```python
from build123d import *

# Parameters (mm, degrees)
EXTRUDE_1_DEPTH           = 20
EXTRUDE_2_DEPTH           = 18.5
EXTRUDE_START             = -6.5
EXTRUDE_8_DEPTH           = 6.5
CUT_EXTRUDE_1_DEPTH       = 3
CUT_EXTRUDE_12_REACH      = 37.343
SKETCH_8_W                = 8
SKETCH_8_H                = 3
SKETCH_1_10_R             = 1.1
CUT_EXTRUDE_13_DEPTH      = 38.032676918
SKETCH_18_W               = 11.552
SKETCH_18_H               = 1
CUT_EXTRUDE_16_DEPTH      = 43.464917168
CHAMFER_1_SIZE            = 4
CHAMFER_1_SIZE2           = 2.309401077
CUT_EXTRUDE_18_REACH      = 39.033
EXTRUDE_START_2           = 3.7
EXTRUDE_9_DEPTH           = 3.7
CUT_EXTRUDE_19_DEPTH      = 11.5
CUT_EXTRUDE_19_DEPTH_BACK = 15.742
SKETCH_22_W               = 16
SKETCH_22_H               = 1.5


with BuildPart() as part:
    # 草图1 → 凸台-拉伸1 (new body)
    with BuildSketch(Plane(origin=(0, 0, 0), x_dir=(1, 0, 0), z_dir=(0, 1, 0))):
        with BuildLine():
            Line((9.493752892, 13.289712364), (-9.506247108, 13.289712364))
            ThreePointArc((-9.506247108, 13.289712364), (-11.274014061, 12.557479317), (-12.006247108, 10.789712364))
            Line((-12.006247108, 10.789712364), (-12.006247108, -10.762287636))
            ThreePointArc((-12.006247108, -10.762287636), (-11.274014061, -12.530054589), (-9.506247108, -13.262287636))
            Line((-9.506247108, -13.262287636), (9.493752892, -13.262287636))
            ThreePointArc((9.493752892, -13.262287636), (11.261519845, -12.530054589), (11.993752892, -10.762287636))
            Line((11.993752892, -10.762287636), (11.993752892, 10.789712364))
            ThreePointArc((11.993752892, 10.789712364), (11.261519845, 12.557479317), (9.493752892, 13.289712364))
        make_face()
        with BuildLine():
            Line((-9.672300027, -7.488904962), (-9.672300027, 7.483095038))
            ThreePointArc((-9.672300027, 7.483095038), (-7.197426293, 8.508221304), (-6.172300027, 10.983095038))
            Line((-6.172300027, 10.983095038), (6.159805812, 10.983095038))
            ThreePointArc((6.159805812, 10.983095038), (7.184932077, 8.508221304), (9.659805812, 7.483095038))
            Line((9.659805812, 7.483095038), (9.659805812, -7.488904962))
            ThreePointArc((9.659805812, -7.488904962), (7.184932077, -8.514031228), (6.159805812, -10.988904962))
            Line((6.159805812, -10.988904962), (-6.172300027, -10.988904962))
            ThreePointArc((-6.172300027, -10.988904962), (-7.197426293, -8.514031228), (-9.672300027, -7.488904962))
        make_face(mode=Mode.SUBTRACT)
    extrude(amount=EXTRUDE_1_DEPTH)

    # 草图3<8> → 凸台-拉伸2 (add)
    with BuildSketch(Plane(origin=(0, 0, 0), x_dir=(1, 0, 0), z_dir=(0, 1, 0))):
        with BuildLine():
            Line((-1.499580884, 4.180163842), (-6.383603139, 9.785400263))
            ThreePointArc((-6.383603139, 9.785400263), (-7.282338381, 8.426127434), (-8.699129058, 7.621110763))
            Line((-8.699129058, 7.621110763), (-3.200900077, 1.310968891))
            ThreePointArc((-3.200900077, 1.310968891), (-2.708791154, -0.002904962), (-3.200900077, -1.316778815))
            Line((-3.200900077, -1.316778815), (-8.699129058, -7.626920687))
            ThreePointArc((-8.699129058, -7.626920687), (-7.282338381, -8.431937358), (-6.383603139, -9.791210187))
            Line((-6.383603139, -9.791210187), (-1.499580884, -4.185973766))
            ThreePointArc((-1.499580884, -4.185973766), (0.01074875, -3.499849106), (1.51940074, -4.189654748))
            Line((1.51940074, -4.189654748), (6.372627583, -9.78704836))
            ThreePointArc((6.372627583, -9.78704836), (7.271462931, -8.43042528), (8.686634842, -7.626920687))
            Line((8.686634842, -7.626920687), (3.188405862, -1.316778815))
            ThreePointArc((3.188405862, -1.316778815), (2.696296938, -0.002904962), (3.188405862, 1.310968891))
            Line((3.188405862, 1.310968891), (8.686634842, 7.621110763))
            ThreePointArc((8.686634842, 7.621110763), (7.271462931, 8.424615355), (6.372627583, 9.781238436))
            Line((6.372627583, 9.781238436), (1.51940074, 4.183844824))
            ThreePointArc((1.51940074, 4.183844824), (0.01074875, 3.494039181), (-1.499580884, 4.180163842))
        make_face()
    extrude(amount=EXTRUDE_2_DEPTH)

    # 草图10 → 凸台-拉伸8 (add)
    with BuildSketch(Plane(origin=(0, 20, 0), x_dir=(1, 0, 0), z_dir=(0, 1, 0)).offset(EXTRUDE_START)):
        with BuildLine():
            Line((-12.006247108, -10.762287636), (-12.006247108, -28.762287636))
            Line((-12.006247108, -28.762287636), (11.993752892, -28.762287636))
            Line((11.993752892, -28.762287636), (11.993752892, -10.762287636))
            ThreePointArc((11.993752892, -10.762287636), (11.261519845, -12.530054589), (9.493752892, -13.262287636))
            Line((9.493752892, -13.262287636), (-9.506247108, -13.262287636))
            ThreePointArc((-9.506247108, -13.262287636), (-11.274014061, -12.530054589), (-12.006247108, -10.762287636))
        make_face()
    extrude(amount=EXTRUDE_8_DEPTH)

    # 草图3<6> → 切除-拉伸1 (cut)
    with BuildSketch(Plane(origin=(0, 0, 0), x_dir=(1, 0, 0), z_dir=(0, 1, 0))):
        with BuildLine():
            Line((-1.499580884, 4.180163842), (-6.383603139, 9.785400263))
            ThreePointArc((-6.383603139, 9.785400263), (-7.282338381, 8.426127434), (-8.699129058, 7.621110763))
            Line((-8.699129058, 7.621110763), (-3.200900077, 1.310968891))
            ThreePointArc((-3.200900077, 1.310968891), (-2.708791154, -0.002904962), (-3.200900077, -1.316778815))
            Line((-3.200900077, -1.316778815), (-8.699129058, -7.626920687))
            ThreePointArc((-8.699129058, -7.626920687), (-7.282338381, -8.431937358), (-6.383603139, -9.791210187))
            Line((-6.383603139, -9.791210187), (-1.499580884, -4.185973766))
            ThreePointArc((-1.499580884, -4.185973766), (0.01074875, -3.499849106), (1.51940074, -4.189654748))
            Line((1.51940074, -4.189654748), (6.372627583, -9.78704836))
            ThreePointArc((6.372627583, -9.78704836), (7.271462931, -8.43042528), (8.686634842, -7.626920687))
            Line((8.686634842, -7.626920687), (3.188405862, -1.316778815))
            ThreePointArc((3.188405862, -1.316778815), (2.696296938, -0.002904962), (3.188405862, 1.310968891))
            Line((3.188405862, 1.310968891), (8.686634842, 7.621110763))
            ThreePointArc((8.686634842, 7.621110763), (7.271462931, 8.424615355), (6.372627583, 9.781238436))
            Line((6.372627583, 9.781238436), (1.51940074, 4.183844824))
            ThreePointArc((1.51940074, 4.183844824), (0.01074875, 3.494039181), (-1.499580884, 4.180163842))
        make_face()
    extrude(amount=CUT_EXTRUDE_1_DEPTH, mode=Mode.SUBTRACT)

    # 草图8 → 切除-拉伸12 (cut, up to next)
    with BuildSketch(Plane.XY.offset(13.262287636), mode=Mode.PRIVATE) as cut_extrude_12_sk1:
        with Locations((0, 1.5)):
            Rectangle(SKETCH_8_W, SKETCH_8_H)
    cut_extrude_12_tool1 = extrude(cut_extrude_12_sk1.sketch, amount=-CUT_EXTRUDE_12_REACH, mode=Mode.PRIVATE) & part.part
    add(cut_extrude_12_tool1.solids().sort_by_distance((0, 1.5, 13.262288))[0], mode=Mode.SUBTRACT)

    # 草图1<10> → 切除-拉伸13 (cut, through all)
    with BuildSketch(Plane(origin=(0, 0, 0), x_dir=(1, 0, 0), z_dir=(0, 1, 0))):
        with Locations(Location((-9.672300027, 10.983095038, 0), (0, 0, 270))):
            Circle(SKETCH_1_10_R)
        with Locations(Location((9.755699973, 10.983095038, 0), (0, 0, 90))):
            Circle(SKETCH_1_10_R)
        with Locations(Location((-9.672300027, -10.988904962, 0), (0, 0, 90))):
            Circle(SKETCH_1_10_R)
        with Locations(Location((9.755699973, -10.988904962, 0), (0, 0, 270))):
            Circle(SKETCH_1_10_R)
    extrude(amount=CUT_EXTRUDE_13_DEPTH, mode=Mode.SUBTRACT)

    # 草图18 → 切除-拉伸16 (cut, through all)
    with BuildSketch(Plane(origin=(11.993752892, 0, 0), x_dir=(0, 0, -1), z_dir=(1, 0, 0))):
        with Locations((1.513712364, 19.5)):
            Rectangle(SKETCH_18_W, SKETCH_18_H)
    extrude(amount=-CUT_EXTRUDE_16_DEPTH, mode=Mode.SUBTRACT)

    # 倒角1
    chamfer_1_edges = [part.edges().sort_by_distance(p)[0] for p in [
        (-0.006247108, 13.5, 28.762287636),
    ]]
    chamfer_1_side = [part.faces().sort_by_distance(p)[0] for p in [
        (-0.006247108, 13.5, 20.952803872),
    ]]
    chamfer(chamfer_1_edges, length=CHAMFER_1_SIZE, length2=CHAMFER_1_SIZE2, reference=chamfer_1_side[0])

    # 切除-拉伸18: up to this plane
    cut_extrude_18_end = Plane(origin=(0, 15.809401077, 28.762287636), z_dir=(0, -0.8660254037844402, 0.49999999999999745))
    # 草图20 → 切除-拉伸18 (cut, up to the surface)
    with BuildSketch(Plane(origin=(0, 20, 0), x_dir=(1, 0, 0), z_dir=(0, 1, 0)), mode=Mode.PRIVATE) as cut_extrude_18_sk1:
        with BuildLine():
            Line((-12.006247108, -26.262287636), (-12.006247108, -28.762287636))
            Line((-12.006247108, -28.762287636), (-9.506247108, -28.762287636))
            ThreePointArc((-9.506247108, -28.762287636), (-11.274014061, -28.030054589), (-12.006247108, -26.262287636))
        make_face()
    cut_extrude_18_tool1 = split(extrude(cut_extrude_18_sk1.sketch, amount=-CUT_EXTRUDE_18_REACH, mode=Mode.PRIVATE), bisect_by=cut_extrude_18_end, keep=Keep.BOTH, mode=Mode.PRIVATE)
    add(cut_extrude_18_tool1.solids().sort_by_distance((-11.447827, 20, 28.203868))[0], mode=Mode.SUBTRACT)
    # 草图20 → 切除-拉伸18 (cut, up to the surface)
    with BuildSketch(Plane(origin=(0, 20, 0), x_dir=(1, 0, 0), z_dir=(0, 1, 0)), mode=Mode.PRIVATE) as cut_extrude_18_sk2:
        with BuildLine():
            Line((11.993752892, -26.262287636), (11.993752892, -28.762287636))
            Line((11.993752892, -28.762287636), (9.493752892, -28.762287636))
            ThreePointArc((9.493752892, -28.762287636), (11.261519845, -28.030054589), (11.993752892, -26.262287636))
        make_face()
    cut_extrude_18_tool2 = split(extrude(cut_extrude_18_sk2.sketch, amount=-CUT_EXTRUDE_18_REACH, mode=Mode.PRIVATE), bisect_by=cut_extrude_18_end, keep=Keep.BOTH, mode=Mode.PRIVATE)
    add(cut_extrude_18_tool2.solids().sort_by_distance((11.435333, 20, 28.203868))[0], mode=Mode.SUBTRACT)

    # 草图21 → 凸台-拉伸9 (add)
    with BuildSketch(Plane(origin=(0, 20, 0), x_dir=(1, 0, 0), z_dir=(0, 1, 0)).offset(EXTRUDE_START_2)):
        with BuildLine():
            ThreePointArc((-9.506247108, -26.730904962), (-11.274014061, -25.998671915), (-12.006247108, -24.230904962))
            Line((-12.006247108, -24.230904962), (-12.006247108, -26.262287636))
            ThreePointArc((-12.006247108, -26.262287636), (-11.274014061, -28.030054589), (-9.506247108, -28.762287636))
            Line((-9.506247108, -28.762287636), (9.493752892, -28.762287636))
            ThreePointArc((9.493752892, -28.762287636), (11.261519845, -28.030054589), (11.993752892, -26.262287636))
            Line((11.993752892, -26.262287636), (11.993752892, -24.230904962))
            ThreePointArc((11.993752892, -24.230904962), (11.261519845, -25.998671915), (9.493752892, -26.730904962))
            Line((9.493752892, -26.730904962), (-9.506247108, -26.730904962))
        make_face()
    extrude(amount=-EXTRUDE_9_DEPTH)

    # 草图22 → 切除-拉伸19 (cut, two sides: drawn at the far end of the back side and taken through both)
    with BuildSketch(Plane(origin=(0, 0, 10.988904962), x_dir=(-1, 0, 0), z_dir=(0, 0, -1)).offset(-CUT_EXTRUDE_19_DEPTH_BACK)):
        with Locations((0.006247108, 19.25)):
            Rectangle(SKETCH_22_W, SKETCH_22_H)
    extrude(amount=CUT_EXTRUDE_19_DEPTH + CUT_EXTRUDE_19_DEPTH_BACK, mode=Mode.SUBTRACT)


solid = part.part
```
Could you check a few things on this model? Use its own coordinates, in mm. A direction names the side the tool comes from. Round coordinates to 2 decimals unless told otherwise and drop trailing zeros. Write each loop counter-clockwise with the first axis right and the second up, starting at its lowest first coordinate (ties: lowest second). Pieces come first, ordered by that corner, then holes. Notation, with made-up numbers: M 49,25.25 L 99,25.25 A26 cw 99,50.25 Z; hole C 86.25,-0.5 d1. An arc over 180 degrees is marked long. Answer in a Markdown table with one row per item. Add a question column.
Q1. On a 3-axis mill with a long thin cutter (end or side, diameter ignored), from which of +Z, -Z, +X, -X, +Y, -Y can I reach the whole of each face in a straight line? I mean faces 4 (the flat face through (-9.672, 10, 0)), 5 (the flat face through (0, 20, -12)), 6 (the flat face through (-11, 19, -1)), 7 (the flat face through (0, 3, 12)), 8 (the flat face through (-8.006, 19, 17)). Say none if no direction works.
Q2. Will these pins go through, and if not, where does the flat tip stop? pin 1 Ø1.8 at (x, z) = (-1, -11.5) entering from +Y; pin 2 Ø1.1 at (y, z) = (1.5, 12) entering from +X; pin 3 Ø0.8 at (x, y) = (-11, 19.5) entering from -Z.
Q3. Imagine slicing it at D-D (y = 22). Please give me the cut outline in (x, z).
Q4. Imagine slicing it at C-C (x = 2.25). Please give me the cut outline in (y, z).
Q5. Imagine slicing it at B-B (x = 5). Please give me the cut outline in (y, z), then the cut area to 3 significant figures.
Q6. If I drill on line 1 (Z direction, x = 5, y = 1); line 2 (X direction, y = 5, z = 0); line 3 (Z direction, x = -6, y = 9.75), over which ranges is the centre line in solid material (lowest first)? Write a range as from..to.
Q7. If we mould it in two halves opening along Z, with no side actions, what happens to faces 1 (the flat face through (3.98, 10.64, -7.02)), 2 (the flat face through (0, 10, -13.29)), 3 (the flat face through (-0.17, 14.67, 26.79))? For each: +Z half, -Z half, draft (parallel to the pull), parting line (faces both ways), or undercut.
Q8. Imagine slicing it at A-A (z = -6). Please give me the cut outline in (x, y).
Values:
| question | item | result |
|---|---|---|
| 1 | face 4 | +Y, -Y |
| 1 | face 5 | -Z, +X, -X, +Y |
| 1 | face 6 | +X, -X, +Y |
| 1 | face 7 | +Z, -Y |
| 1 | face 8 | +Y |
| 2 | pin 1 | y = 20 |
| 2 | pin 2 | x = 11.9 |
| 2 | pin 3 | z = -13.04 |
| 3 | outline | M -12.01,24.23 A2.5 cw -9.51,26.73 L 9.49,26.73 A2.5 cw 11.99,24.23 L 11.99,26.26 A2.5 ccw 9.49,28.76 L -9.51,28.76 A2.5 ccw -12.01,26.26 Z |
| 4 | outline | M 0,-13.29 L 20,-13.29 L 20,-10.98 L 0,-10.98 Z; M 3,-5.03 L 18.5,-5.03 L 18.5,5.03 L 3,5.03 Z; M 3,10.99 L 18.5,10.99 L 18.5,26.73 L 23.7,26.73 L 23.7,28.76 L 15.81,28.76 L 13.5,24.76 L 13.5,13.26 L 3,13.26 Z |
| 5 | outline | M 0,-13.29 L 20,-13.29 L 20,-10.98 L 0,-10.98 Z; M 0,10.99 L 18.5,10.99 L 18.5,26.73 L 23.7,26.73 L 23.7,28.76 L 15.81,28.76 L 13.5,24.76 L 13.5,13.26 L 0,13.26 Z; M 3,-8.2 L 18.5,-8.2 L 18.5,-3.39 L 3,-3.39 Z; M 3,3.4 L 18.5,3.4 L 18.5,8.2 L 3,8.2 Z |
| 5 | area | 321 mm^2 |
| 6 | line 1 | -13.29..-10.98, 10.99..13.26 |
| 6 | line 2 | -12.01..-9.67, -2.71..2.7, 9.66..11.99 |
| 6 | line 3 | -13.29..-10.98, -9.35..-4.52, 4.53..9.35, 10.99..13.26 |
| 7 | face 1 | undercut |
| 7 | face 2 | -Z half |
| 7 | face 3 | +Z half |
| 8 | outline | M -12.01,0 L -9.67,0 L -9.67,19 L -12.01,19 Z; M -7.29,3 L -3.09,3 L -3.09,18.5 L -7.29,18.5 Z; M 3.09,3 L 7.27,3 L 7.27,18.5 L 3.09,18.5 Z; M 9.66,0 L 11.99,0 L 11.99,19 L 9.66,19 Z |
